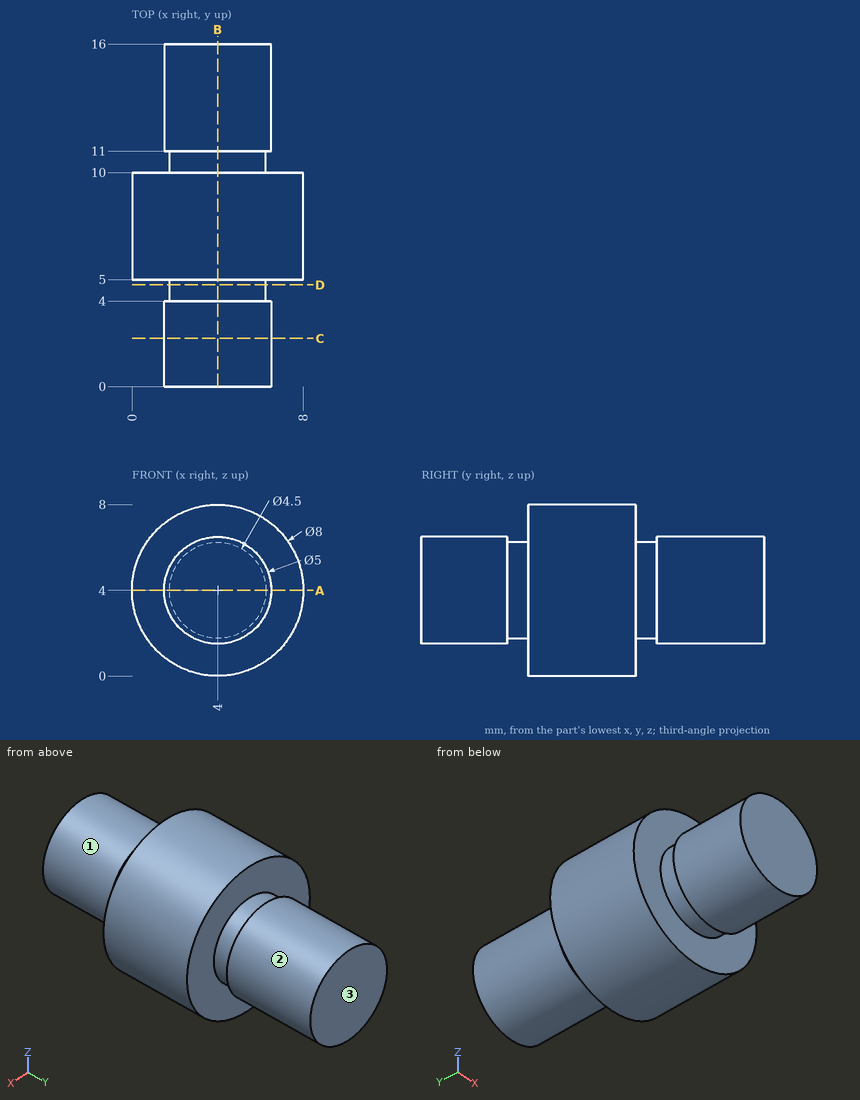
Study the drawing (mm; zero at the part's minimum x, y, z) and answer. A direction names the side the tool comes from. Give positions to 0.01 mm unless a question says otherwise; leave off trailing zeros. Write each loop counter-clockwise with the first axis right and the second up, starting at its lowest first coordinate (ties: lowest second). Pieces come first, ordered by that corner, then holes. Notation, with made-up numbers: M 28,47 L 38,47 A21 ccw 38,63 Z; hole C 5.5,23.25 d5. An arc over 180 degrees is marked long. Put each result on its own line as item: value. Start each with the question number.
1. Which of the six approach directions +Z, -Z, +X, -X, +Y, -Y give full straight-line access (tool end or side, diameter ignored) to the marked faces 1, 2 and 3?
2. The part is cut by section B-B, the plane x = 4. Give the vertices of the cut face in (y, z), and give its area (3 significant figures).
3. The part is cut by section A-A, the plane z = 4. Give the vertices of the cut face in (x, y), and give its area (3 significant figures).
4. The part is cut by section D-D, the plane y = 4.75. Give the vertices of the cut face in (x, z).
5. Consider line 1 along Y through (x, z) = (0.5, 5); line 2 along X through (y, z) = (9.25, 0.5); line 3 along Z through (x, y) = (2.5, 7.25). Determine where each line is inside the solid, lowest interval first.
6. Each of these flat-tipped pins is pushed along its axis until it touches: pin 1 Ø4 at (x, z) = (4, 5) entering from -Y; pin 2 Ø1.5 at (x, y) = (4, 4) entering from -Z; pin 3 Ø1.5 at (y, z) = (2.5, 5) entering from +X; pin 4 Ø1.5 at (x, y) = (2, 4.5) entering from -Z. Where does it stop, or does it pass through?
7. The part is cut by section C-C, the plane y = 2.25. Give the vertices of the cut face in (x, z).
Final values:
1. face 1: -Y
1. face 2: +Y
1. face 3: +Z, -Z, +X, -X, +Y
2. outline: M 0,1.5 L 4,1.5 L 4,1.75 L 5,1.75 L 5,0 L 10,0 L 10,1.75 L 11,1.75 L 11,1.5 L 16,1.5 L 16,6.5 L 11,6.5 L 11,6.25 L 10,6.25 L 10,8 L 5,8 L 5,6.25 L 4,6.25 L 4,6.5 L 0,6.5 Z
2. area: 94.0 mm²
3. outline: M 0,5 L 1.75,5 L 1.75,4 L 1.5,4 L 1.5,0 L 6.5,0 L 6.5,4 L 6.25,4 L 6.25,5 L 8,5 L 8,10 L 6.25,10 L 6.25,11 L 6.5,11 L 6.5,16 L 1.5,16 L 1.5,11 L 1.75,11 L 1.75,10 L 0,10 Z
3. area: 94.0 mm²
4. outline: C 4,4 d4.5
5. line 1: y = 5 to 10
5. line 2: x = 2.06 to 5.94
5. line 3: z = 0.29 to 7.71
6. pin 1: stops at y = 0
6. pin 2: stops at z = 1.5
6. pin 3: stops at x = 6.49
6. pin 4: stops at z = 0.27
7. outline: C 4,4 d5
